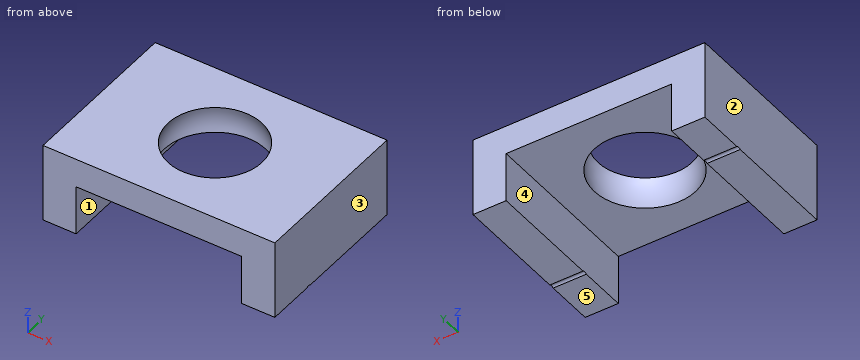
```python
from build123d import *

# Parameters (mm, degrees)
BOX006_W                = 21
BOX006_H                = 17
BOX006_DEPTH            = 12
CYLINDER005_R           = 2.5
CYLINDER005_DEPTH       = 10
CYLINDER004_R           = 0.25
CYLINDER004_DEPTH       = 10
CYLINDER004_PITCH_ANGLE = 90
CYLINDER003_R           = 0.25
CYLINDER003_DEPTH       = 10
CYLINDER003_PITCH_ANGLE = 90
BOX002_W                = 6.5
BOX002_H                = 4.8
BOX002_DEPTH            = 1
BOX003_W                = 10
BOX003_H                = 12
BOX003_DEPTH            = 3
BOX001_W                = 14
BOX001_H                = 10
BOX001_DEPTH            = 7.25


with BuildPart() as cube006:
    # Box006 → Box006 (new body)
    with BuildSketch(Plane(origin=(-9, -7, -3.5), x_dir=(1, 0, 0), z_dir=(0, 0, 1))):
        with Locations((10.5, 8.5)):
            Rectangle(BOX006_W, BOX006_H)
    extrude(amount=BOX006_DEPTH)


with BuildPart() as cylinder005:
    # Cylinder005 → Cylinder005 (new body)
    with BuildSketch(Plane.XY.offset(0.5)):
        Circle(CYLINDER005_R)
    extrude(amount=CYLINDER005_DEPTH)


with BuildPart() as fusion004:
    # Sphere001 → Sphere001 (revolve)
    with BuildSketch(Plane.XZ):
        with BuildLine():
            ThreePointArc((0, -3.1), (3.1, 0), (0, 3.1))
            Line((0, 3.1), (0, -3.1))
        make_face()
    revolve(axis=Axis((0, 0, 0), (0, 0, 1)))

    # Fusion004: union Cylinder005
    add(cylinder005.part)


with BuildPart() as cylinder004:
    # Cylinder004 → Cylinder004 (new body)
    with BuildSketch(Plane.XY):
        Circle(CYLINDER004_R)
    extrude(amount=CYLINDER004_DEPTH)


with BuildPart() as cylinder004_1:
    # Cylinder004 pitch: moved
    add(cylinder004.part.rotate(Axis((0, 0, 0), (0, 1, 0)), CYLINDER004_PITCH_ANGLE))


with BuildPart() as cylinder004_2:
    # Cylinder004 placement: moved
    add(cylinder004_1.part.moved(Location((0, -2, -3.7))))


with BuildPart() as fusion:
    # Cylinder003 → Cylinder003 (new body)
    with BuildSketch(Plane.XY):
        Circle(CYLINDER003_R)
    extrude(amount=CYLINDER003_DEPTH)


with BuildPart() as fusion_1:
    # Cylinder003 pitch: moved
    add(fusion.part.rotate(Axis((0, 0, 0), (0, 1, 0)), CYLINDER003_PITCH_ANGLE))


with BuildPart() as fusion_2:
    # Cylinder003 placement: moved
    add(fusion_1.part.moved(Location((-11, 2, -3.7))))

    # Fusion: union Cylinder004
    add(cylinder004_2.part)


with BuildPart() as fusion001:
    # Box002 → Box002 (new body)
    with BuildSketch(Plane(origin=(-3.25, -2.4, -4.2), x_dir=(1, 0, 0), z_dir=(0, 0, 1))):
        with Locations((3.25, 2.4)):
            Rectangle(BOX002_W, BOX002_H)
    extrude(amount=BOX002_DEPTH)

    # Fusion001: union Fusion
    add(fusion_2.part)


with BuildPart() as cube003:
    # Box003 → Box003 (new body)
    with BuildSketch(Plane(origin=(-5, -6, -3.5), x_dir=(1, 0, 0), z_dir=(0, 0, 1))):
        with Locations((5, 6)):
            Rectangle(BOX003_W, BOX003_H)
    extrude(amount=BOX003_DEPTH)


with BuildPart() as ball_and_screw_holder:
    # Box001 → Box001 (new body)
    with BuildSketch(Plane(origin=(-7, -5, -6), x_dir=(1, 0, 0), z_dir=(0, 0, 1))):
        with Locations((7, 5)):
            Rectangle(BOX001_W, BOX001_H)
    extrude(amount=BOX001_DEPTH)

    # Cut: cut Cube003
    add(cube003.part, mode=Mode.SUBTRACT)

    # Cut001: cut Fusion001
    add(fusion001.part, mode=Mode.SUBTRACT)

    # Cut002: cut Fusion004
    add(fusion004.part, mode=Mode.SUBTRACT)

    # Common: intersect Cube006
    add(cube006.part, mode=Mode.INTERSECT)


solid = ball_and_screw_holder.part
```
The listing builds one solid part. Answer for the finished solid, in the listing's coordinates (mm). Face numbers are marked on the shaded views. A direction names the side the tool comes from. Coordinates: 2 decimals unless noted, no trailing zeros. Write each loop counter-clockwise with the first axis right and the second up, starting at its lowest first coordinate (ties: lowest second). Pieces come first, ordered by that corner, then holes. Notation, with made-up numbers: (61.25, 46) - (71.25, 46) arc R10 cw to (71.25, 62) - close; hole circle Ø3 at (35, 25). An arc over 180 degrees is marked (long way). Return JSON: item names as keys, results as strings. Group by question number.
1. A cutting plane is placed at C-C, the plane z = -1.05. Determine the outline of the cut face in (x, y), plus the area to 3 significant figures.
2. Straight lines are drawn through the part: L1, parallel to X at y = 2.5, z = -2.65; L2, parallel to Y at x = 0, z = 0.15; L3, parallel to Z at x = 4.5, y = 2.25. For each, find the intervals that lie inside material, in ascending order.
3. A cutting plane is placed at B-B, the plane y = 0.25. Determine the outline of the cut face in (x, z).
4. A cutting plane is placed at A-A, the plane x = 2.25. Determine the outline of the cut face in (y, z), plus the area to 3 significant figures.
5. Determine the mould class of the marked faces 3, 4 and 5 for opening direction X: released by +X, released by -X, zero draft, split by the parting line, or undercut.
6. A cutting plane is placed at D-D, the plane y = -3.75. Determine the outline of the cut face in (x, z).
7. Which of the six approach directions +Z, -Z, +X, -X, +Y, -Y give full straight-line access (tool end or side, diameter ignored) to the marked faces 1 and 2?
8. Given pin 1 (1 mm diameter, centred on x = 1.5, y = 3.5, fed in from -Z), flat-ended and moving along its own axis, determine where the tip first touches the part or whether it passes through.
Ans:
{
 "1": {"outline": "(-7, -5) - (-5, -5) - (-5, 5) - (-7, 5) - close; (5, -5) - (7, -5) - (7, 5) - (5, 5) - close", "area": "40.0 mm²"},
 "2": {"L1": "-7 to -5, 5 to 7", "L2": "-5 to -3.1, 3.1 to 5", "L3": "-0.5 to 1.25"},
 "3": {"outline": "(-7, -3.5) - (-5, -3.5) - (-5, -0.5) - (-3.05, -0.5) arc R3.09 cw to (-2.83, 1.25) - (-7, 1.25) - close; (2.83, 1.25) arc R3.09 cw to (3.05, -0.5) - (5, -0.5) - (5, -3.5) - (7, -3.5) - (7, 1.25) - close"},
 "4": {"outline": "(-5, -0.5) - (-2.07, -0.5) arc R2.13 cw to (-1.73, 1.25) - (-5, 1.25) - close; (1.73, 1.25) arc R2.13 cw to (2.07, -0.5) - (5, -0.5) - (5, 1.25) - close", "area": "10.4 mm²"},
 "5": {"face 3": "released by +X", "face 4": "undercut", "face 5": "zero draft"},
 "6": {"outline": "(-7, -3.5) - (-5, -3.5) - (-5, -0.5) - (5, -0.5) - (5, -3.5) - (7, -3.5) - (7, 1.25) - (-7, 1.25) - close"},
 "7": {"face 1": "-Z, +Y, -Y", "face 2": "+Z, -Z, -X, +Y, -Y"},
 "8": {"pin 1": "z = -0.5"}
}
